Design review of the part built by this model. Coordinates are the model's own, in mm. Coordinates: 2 decimals unless noted, no trailing zeros. Answer in a Markdown table with one row per item.
from build123d import *

# Parameters (mm, degrees)
SKETCH1_W           = 25
SKETCH1_H           = 25
SKETCH1_R           = 0.55
BOSS_EXTRUDE1_DEPTH = 10


with BuildPart() as part:
    # Sketch1 → Boss-Extrude1 (new body)
    with BuildSketch(Plane(origin=(0, 0, 0), x_dir=(1, 0, 0), z_dir=(0, 1, 0))):
        Rectangle(SKETCH1_W, SKETCH1_H)
        with Locations((-8.5, 8.5)):
            Circle(SKETCH1_R, mode=Mode.SUBTRACT)
        with Locations((-6.15, 8.5)):
            Circle(SKETCH1_R, mode=Mode.SUBTRACT)
        with Locations((-3.8, 8.5)):
            Circle(SKETCH1_R, mode=Mode.SUBTRACT)
        with Locations((-1.45, 8.5)):
            Circle(SKETCH1_R, mode=Mode.SUBTRACT)
        with Locations((0.9, 8.5)):
            Circle(SKETCH1_R, mode=Mode.SUBTRACT)
        with Locations((3.25, 8.5)):
            Circle(SKETCH1_R, mode=Mode.SUBTRACT)
        with Locations((5.6, 8.5)):
            Circle(SKETCH1_R, mode=Mode.SUBTRACT)
        with Locations((7.95, 8.5)):
            Circle(SKETCH1_R, mode=Mode.SUBTRACT)
        with Locations((-6.15, 6.15)):
            Circle(SKETCH1_R, mode=Mode.SUBTRACT)
        with Locations((-3.8, 6.15)):
            Circle(SKETCH1_R, mode=Mode.SUBTRACT)
        with Locations((-1.45, 6.15)):
            Circle(SKETCH1_R, mode=Mode.SUBTRACT)
        with Locations((0.9, 6.15)):
            Circle(SKETCH1_R, mode=Mode.SUBTRACT)
        with Locations((3.25, 6.15)):
            Circle(SKETCH1_R, mode=Mode.SUBTRACT)
        with Locations((5.6, 6.15)):
            Circle(SKETCH1_R, mode=Mode.SUBTRACT)
        with Locations((7.95, 6.15)):
            Circle(SKETCH1_R, mode=Mode.SUBTRACT)
        with Locations((-6.15, 3.8)):
            Circle(SKETCH1_R, mode=Mode.SUBTRACT)
        with Locations((-3.8, 3.8)):
            Circle(SKETCH1_R, mode=Mode.SUBTRACT)
        with Locations((-1.45, 3.8)):
            Circle(SKETCH1_R, mode=Mode.SUBTRACT)
        with Locations((0.9, 3.8)):
            Circle(SKETCH1_R, mode=Mode.SUBTRACT)
        with Locations((3.25, 3.8)):
            Circle(SKETCH1_R, mode=Mode.SUBTRACT)
        with Locations((5.6, 3.8)):
            Circle(SKETCH1_R, mode=Mode.SUBTRACT)
        with Locations((7.95, 3.8)):
            Circle(SKETCH1_R, mode=Mode.SUBTRACT)
        with Locations((-6.15, 1.45)):
            Circle(SKETCH1_R, mode=Mode.SUBTRACT)
        with Locations((-3.8, 1.45)):
            Circle(SKETCH1_R, mode=Mode.SUBTRACT)
        with Locations((-1.45, 1.45)):
            Circle(SKETCH1_R, mode=Mode.SUBTRACT)
        with Locations((0.9, 1.45)):
            Circle(SKETCH1_R, mode=Mode.SUBTRACT)
        with Locations((3.25, 1.45)):
            Circle(SKETCH1_R, mode=Mode.SUBTRACT)
        with Locations((5.6, 1.45)):
            Circle(SKETCH1_R, mode=Mode.SUBTRACT)
        with Locations((7.95, 1.45)):
            Circle(SKETCH1_R, mode=Mode.SUBTRACT)
        with Locations((-6.15, -0.9)):
            Circle(SKETCH1_R, mode=Mode.SUBTRACT)
        with Locations((-3.8, -0.9)):
            Circle(SKETCH1_R, mode=Mode.SUBTRACT)
        with Locations((-1.45, -0.9)):
            Circle(SKETCH1_R, mode=Mode.SUBTRACT)
        with Locations((0.9, -0.9)):
            Circle(SKETCH1_R, mode=Mode.SUBTRACT)
        with Locations((3.25, -0.9)):
            Circle(SKETCH1_R, mode=Mode.SUBTRACT)
        with Locations((5.6, -0.9)):
            Circle(SKETCH1_R, mode=Mode.SUBTRACT)
        with Locations((7.95, -0.9)):
            Circle(SKETCH1_R, mode=Mode.SUBTRACT)
        with Locations((-6.15, -3.25)):
            Circle(SKETCH1_R, mode=Mode.SUBTRACT)
        with Locations((-3.8, -3.25)):
            Circle(SKETCH1_R, mode=Mode.SUBTRACT)
        with Locations((-1.45, -3.25)):
            Circle(SKETCH1_R, mode=Mode.SUBTRACT)
        with Locations((0.9, -3.25)):
            Circle(SKETCH1_R, mode=Mode.SUBTRACT)
        with Locations((3.25, -3.25)):
            Circle(SKETCH1_R, mode=Mode.SUBTRACT)
        with Locations((5.6, -3.25)):
            Circle(SKETCH1_R, mode=Mode.SUBTRACT)
        with Locations((7.95, -3.25)):
            Circle(SKETCH1_R, mode=Mode.SUBTRACT)
        with Locations((-6.15, -5.6)):
            Circle(SKETCH1_R, mode=Mode.SUBTRACT)
        with Locations((-3.8, -5.6)):
            Circle(SKETCH1_R, mode=Mode.SUBTRACT)
        with Locations((-1.45, -5.6)):
            Circle(SKETCH1_R, mode=Mode.SUBTRACT)
        with Locations((0.9, -5.6)):
            Circle(SKETCH1_R, mode=Mode.SUBTRACT)
        with Locations((3.25, -5.6)):
            Circle(SKETCH1_R, mode=Mode.SUBTRACT)
        with Locations((5.6, -5.6)):
            Circle(SKETCH1_R, mode=Mode.SUBTRACT)
        with Locations((7.95, -5.6)):
            Circle(SKETCH1_R, mode=Mode.SUBTRACT)
        with Locations((-6.15, -7.95)):
            Circle(SKETCH1_R, mode=Mode.SUBTRACT)
        with Locations((-3.8, -7.95)):
            Circle(SKETCH1_R, mode=Mode.SUBTRACT)
        with Locations((-1.45, -7.95)):
            Circle(SKETCH1_R, mode=Mode.SUBTRACT)
        with Locations((0.9, -7.95)):
            Circle(SKETCH1_R, mode=Mode.SUBTRACT)
        with Locations((3.25, -7.95)):
            Circle(SKETCH1_R, mode=Mode.SUBTRACT)
        with Locations((5.6, -7.95)):
            Circle(SKETCH1_R, mode=Mode.SUBTRACT)
        with Locations((7.95, -7.95)):
            Circle(SKETCH1_R, mode=Mode.SUBTRACT)
        with Locations((-8.5, 6.15)):
            Circle(SKETCH1_R, mode=Mode.SUBTRACT)
        with Locations((-8.5, 3.8)):
            Circle(SKETCH1_R, mode=Mode.SUBTRACT)
        with Locations((-8.5, 1.45)):
            Circle(SKETCH1_R, mode=Mode.SUBTRACT)
        with Locations((-8.5, -0.9)):
            Circle(SKETCH1_R, mode=Mode.SUBTRACT)
        with Locations((-8.5, -3.25)):
            Circle(SKETCH1_R, mode=Mode.SUBTRACT)
        with Locations((-8.5, -5.6)):
            Circle(SKETCH1_R, mode=Mode.SUBTRACT)
        with Locations((-8.5, -7.95)):
            Circle(SKETCH1_R, mode=Mode.SUBTRACT)
    extrude(amount=BOSS_EXTRUDE1_DEPTH)


solid = part.part
(1) Add section A-A, the plane z = 3.25. Give the number of separate pieces and of enclosed holes in the cut face, and give its area (3 significant figures).
Return value:
| item | result |
|---|---|
| separate pieces | 9 |
| enclosed holes | 0 |
| area | 162 mm2 |
(2) Insertion check: pin 1 Ø0.7 at (x, z) = (-1.45, 3.25) entering from +Y; pin 2 Ø12 at (x, z) = (-1.5, 6.5) entering from -Y. Each pin has a flat end and moves straight along its axis. Give the tip position at first contact, or say it passes through.
Return value:
| item | result |
|---|---|
| pin 1 | passes through |
| pin 2 | stops at y = 0 |
(3) Draft analysis for pull direction Z (two halves, no side actions). For faces 1 (the flat face through (0, 10, 0)), 2 (the cylindrical face through (-5.9, 4.93, -3.31)), state which applies: pulls with the +Z half, pulls with the -Z half, needs draft (parallel to the pull), parting line crosses it, or undercut.
Return value:
| item | result |
|---|---|
| face 1 | needs draft |
| face 2 | undercut |
